Autodesk Inventor part; units mm, degrees
ref_plane "YZ Plane" through (0, 0, 0) normal (1, 0, 0) x (0, 1, 0)
ref_plane "XZ Plane" through (0, 0, 0) normal (0, 1, 0) x (-1, 0, 0)
ref_plane "XY Plane" through (0, 0, 0) normal (0, 0, 1) x (1, 0, 0)
sketch "Sketch2" plane through (0, 0, 0) normal (0, 1, 0) x (-1, 0, 0)
  line L0 (2, -40) -> (-2, -40)
  line L1 (-2, -40) -> (-2, 40)
  line L2 (-2, 40) -> (2, 40)
  line L3 (2, 40) -> (2, -40)
  line L4 (44, -2) -> (-44, -2)
  line L5 (-44, -2) -> (-44, 2)
  line L6 (-44, 2) -> (44, 2)
  line L7 (44, 2) -> (44, -2)
  line L8 (44, 5) -> (-44, 5)
  line L9 (-44, 5) -> (-44, -5)
  line L10 (-44, -5) -> (44, -5)
  line L11 (44, -5) -> (44, 5)
  point P0 (0, 0)
  point P1 (0, -40)
  point P2 (-44, 0)
  point P3 (0, -2)
  point P4 (-2, 0)
  point P5 (2, 2)
  point P6 (-2, 2)
  point P7 (-2, -2)
  point P8 (2, -2)
  point P9 (44, 0)
  dimension "d0" = 4
  dimension "d1" = 4
  dimension "d2" = 80
  dimension "d3" = 88
  dimension "d6" = 10
extrude "Extrusion1" add sketch "Sketch2" along normal blind 30 contours L0 L1 L10 L3 | L10 L1 L4 L3 | L4 L1 L6 L3 | L3 L6 L7 L4 | L4 L5 L6 L1 | L6 L1 L8 L3 | L8 L1 L2 L3
extrude "Extrusion2" add sketch "Sketch2" against normal blind 1.5 contours L10 L1 L4 L3 | L3 L4 L11 L10 | L10 L9 L4 L1 | L4 L1 L6 L3 | L3 L6 L7 L4 | L4 L5 L6 L1 | L6 L1 L8 L3 | L3 L8 L11 L6 | L6 L9 L8 L1
properties part number "halfdrawerdivider"
Design review of the part built by this model. Coordinates are the model's own, in mm. A direction names the side the tool comes from. Coordinates: 2 decimals unless noted, no trailing zeros. Order: outer loops, then holes, each group sorted by start corner. A loop starts at its lowest first (then second) coordinate and runs counter-clockwise, first axis right, second up. Notation, with made-up numbers: (24.5, 84) -> (47.5, 84) arc R22 cw to (47.5, 115) -> close; hole circle Ø3 at (-28.75, 16.5). An arc over 180 degrees is marked (long way). One line per item, written item: value.
1) To check wall thickness, follow probe 1 along Z at (x, y) = (27, 2.5); probe 2 along Y at (x, z) = (-1, -28). State the ranges of each line that lie inside material, in increasing order. Write a range as [from, to].
Output values:
probe 1: z = [-2, 2]
probe 2: y = [0, 30]
2) We need section A-A, the plane x = 13.5. Give the boundary of the cut face in (y, z), then the cut area to 3 significant figures.
Output values:
outline: (-1.5, -5) -> (0, -5) -> (0, -2) -> (30, -2) -> (30, 2) -> (0, 2) -> (0, 5) -> (-1.5, 5) -> close
area: 135 mm2
3) We need section C-C, the plane y = 17. Give the boundary of the cut face in (x, z).
Output values:
outline: (-44, -2) -> (-2, -2) -> (-2, -40) -> (2, -40) -> (2, -2) -> (44, -2) -> (44, 2) -> (2, 2) -> (2, 40) -> (-2, 40) -> (-2, 2) -> (-44, 2) -> close
4) We need section D-D, the plane z = 10. Give the boundary of the cut face in (x, y), then the cut area to 3 significant figures.
Output values:
outline: (-2, 0) -> (2, 0) -> (2, 30) -> (-2, 30) -> close
area: 120 mm2
5) Machinability: for faces 1 (the face through (-23, 0, -3)), 2 (the face through (0, 0, 23)), 3 (the face through (23, 0, -3)), 4 (the face through (0, 0, -22)), 5 (the face through (23, 0, 4)), which of the approach directions +Z, -Z, +X, -X, +Y, -Y give a long, thin tool a straight path to every point of the face, cutting with its end or side? Answer none if there is none.
Output values:
face 1: -Z, -X, +Y
face 2: +Z, +X, -X, -Y
face 3: -Z, +X, +Y
face 4: -Z, +X, -X, -Y
face 5: +Z, +X, +Y
6) We need section B-B, the plane z = -3.5. Give the boundary of the cut face in (x, y), then the cut area to 3 significant figures.
Output values:
outline: (-44, -1.5) -> (44, -1.5) -> (44, 0) -> (2, 0) -> (2, 30) -> (-2, 30) -> (-2, 0) -> (-44, 0) -> close
area: 252 mm2
7) Clearance check with flat-ended pins moving along their axes: P1, Ø1.2, axis at x = 0, z = 19.5, coming from the -Y side; P2, Ø1, axis at x = 8, y = 8, coming from the -Z side; P3, Ø9, axis at x = 19.5, y = 17, coming from the +Z side. State where each tip first meets the part, or that it passes through.
Output values:
P1: stops at y = 0
P2: stops at z = -2
P3: stops at z = 2
